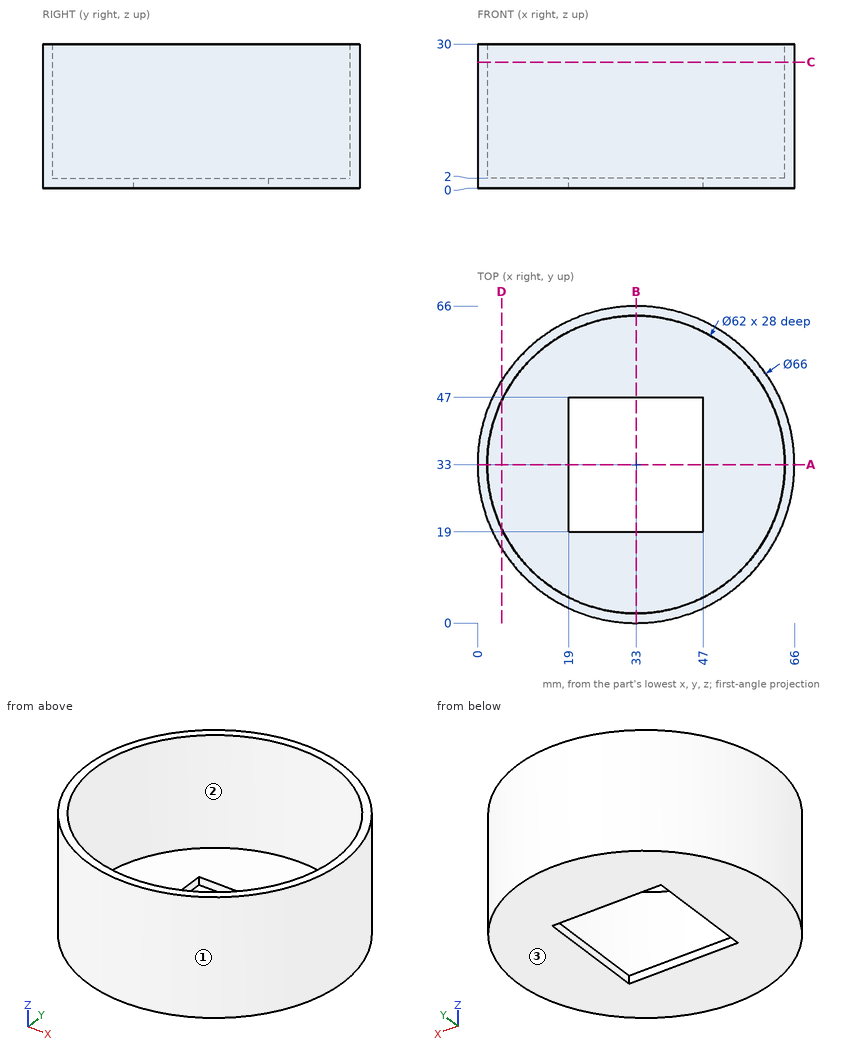
Answer from the drawing. Dimensions are ordinates in mm from the lowest x, y and z of the part. Give positions to 0.01 mm unless a question says otherwise; leave off trailing zeros. Order: outer loops, then holes, each group sorted by start corner. A loop starts at its lowest first (then second) coordinate and runs counter-clockwise, first axis right, second up. Notation, with made-up numbers: (-7, -10) -> (-1, -10) arc R28 cw to (-1, 28) -> close; hole circle Ø7 at (80.25, 80). An arc over 180 degrees is marked (long way). One line per item, written item: value.
Item 1: Find section C-C, the plane z = 26.25. Give the vertices of the cut face in (x, y).
Answer sheet:
outline: circle Ø66 at (33, 33); hole circle Ø62 at (33, 33)
Item 2: Flat-ended cylindrical pins translate along their axes: P1, Ø10, axis at x = 53, z = 11, coming from the -Y side; P2, Ø18.5, axis at x = 39.5, y = 45.5, coming from the +Z side; P3, Ø5, axis at y = 59, z = 8.5, coming from the +X side. Find the tip coordinate at first contact, or state that the pin passes through.
Answer sheet:
P1: y = 3.61
P2: z = 2
P3: x = 56.17
Item 3: Straight lines are drawn through the part: probe 1 along Y at (x, z) = (33, 8.5); probe 2 along Z at (x, y) = (14, 45); probe 3 along X at (y, z) = (34, 5). For each, find the intervals that lie inside material, in ascending order.
Answer sheet:
probe 1: 0 to 2, 64 to 66
probe 2: 0 to 2
probe 3: 0.02 to 2.02, 63.98 to 65.98
Item 4: Find section D-D, the plane x = 5. Give the vertices of the cut face in (y, z), plus the area to 3 significant figures.
Answer sheet:
outline: (15.54, 0) -> (50.46, 0) -> (50.46, 30) -> (46.3, 30) -> (46.3, 2) -> (19.7, 2) -> (19.7, 30) -> (15.54, 30) -> close
area: 303 mm²
Item 5: Determine the mould class of the marked faces 1, 2 and 3 for opening direction Y: released by +Y, released by -Y, zero draft, split by the parting line, or undercut.
Answer sheet:
face 1: split by the parting line
face 2: undercut
face 3: zero draft
Item 6: Find section A-A, the plane y = 33. Give the vertices of the cut face in (x, z), plus the area to 3 significant figures.
Answer sheet:
outline: (0, 0) -> (19, 0) -> (19, 2) -> (2, 2) -> (2, 30) -> (0, 30) -> close; (47, 0) -> (66, 0) -> (66, 30) -> (64, 30) -> (64, 2) -> (47, 2) -> close
area: 188 mm²
